Verification items for the finished model (mm, model axes). Face numbers are marked on the shaded views. A direction names the side the tool comes from. Round coordinates to 2 decimals unless told otherwise and drop trailing zeros. Order: outer loops, then holes, each group sorted by start corner. A loop starts at its lowest first (then second) coordinate and runs counter-clockwise, first axis right, second up. Notation, with made-up numbers: M 54.25,73.5 L 85.25,73.5 A4 cw 85.25,77.5 Z; hole C 8,29.25 d3. An arc over 180 degrees is marked long. Use one line per item in the form item = value. Start each with the question number.
Item 1: Thickness scan on probe 1 along Y at (x, z) = (0, 0.7); probe 2 along X at (y, z) = (0.75, 0.55); probe 3 along Z at (x, y) = (1.75, -4.5). Record the ranges inside material, lowest first. Write a range as [from, to].
Item 2: Cross-section at A-A on y = 0. Enter the section's corners in (x, z) (3 decimals).
Item 3: Cross-section at D-D on z = 0.2. Enter the section's corners in (x, y).
Item 4: Go/stop test with a flat-tipped pin: pin 1 Ø3 at (x, y) = (0, 0) entering from -Z. Record where the tip stops, or that it passes through.
Item 5: Cross-section at C-C on y = -1.5. Enter the section's corners in (x, z) (3 decimals).
Item 6: Tool access check on the marked faces 1, 2, 3, 4 and 5. Record the directions out of +Z, -Z, +X, -X, +Y, -Y that give a thin tool (end or side, any length) a straight path to the whole face; none if there is none.
Item 7: Cross-section at B-B on z = 1.75. Enter the section's corners in (x, y) (3 decimals).
from build123d import *

# Parameters (mm, degrees)
F0_R          = 5.2
F1_DEPTH      = 1
F2_R          = 2
F3_DEPTH      = 1.48
F4_DEPTH      = 25
F4_DEPTH_BACK = 25
F5_R          = 0.1


with BuildPart() as f1:
    # F0 (on Top) → F1 (new body)
    with BuildSketch(Plane.XY):
        Circle(F0_R)
    extrude(amount=F1_DEPTH)

    # F2 (on face) → F3 (join)
    with BuildSketch(Plane.XY.offset(1)):
        Polygon((3.575, -2.064027), (3.575, 2.064027), (0, 4.128054), (-3.575, 2.064027), (-3.575, -2.064027), (0, -4.128054), align=None)
        Circle(F2_R, mode=Mode.SUBTRACT)
    extrude(amount=F3_DEPTH)

    # F2 (on face) → F4 (cut, two sides)
    with BuildSketch(Plane.XY.offset(1)) as f4_sk:
        Circle(F2_R)
    extrude(amount=-F4_DEPTH, mode=Mode.SUBTRACT)
    extrude(f4_sk.sketch, amount=-F4_DEPTH_BACK, mode=Mode.SUBTRACT)

    # F5
    f5_edges = [f1.edges().sort_by_distance(p)[0] for p in [
        (1.7875, -3.096041, 2.48),
        (3.575, 0, 2.48),
        (-1.7875, -3.096041, 2.48),
        (-3.575, 0, 2.48),
        (-1.7875, 3.096041, 2.48),
        (1.7875, 3.096041, 2.48),
    ]]
    fillet(f5_edges, radius=F5_R)


solid = f1.part
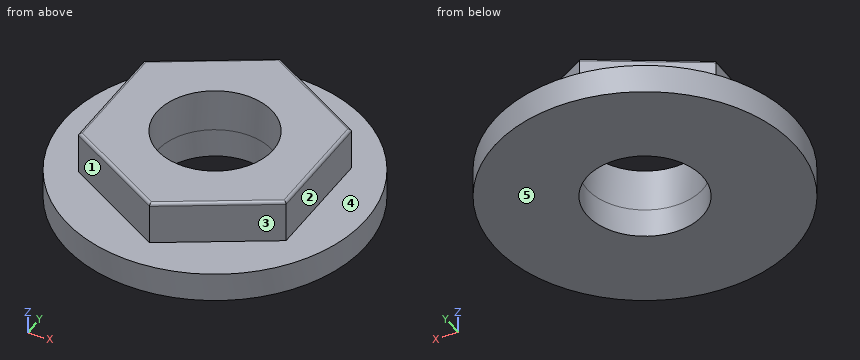
Output values:
q1.probe_1 = [-5.2, -2], [2, 5.2]
q1.probe_2 = [-5.15, -1.85], [1.85, 5.15]
q1.probe_3 = [0, 1]
q2.outline = M -5.2,0 L -2,0 L -2,2.48 L -3.475,2.48 A0.1 ccw -3.575,2.38 L -3.575,1 L -5.2,1 Z; M 2,0 L 5.2,0 L 5.2,1 L 3.575,1 L 3.575,2.38 A0.1 ccw 3.475,2.48 L 2,2.48 Z
q3.outline = C 0,0 d10.4; hole C 0,0 d4
q4.pin_1 = through
q5.outline = M -4.979,0 L -1.323,0 L -1.323,2.48 L -3.475,2.48 A0.1 ccw -3.575,2.38 L -3.575,1 L -4.979,1 Z; M 1.323,0 L 4.979,0 L 4.979,1 L 3.575,1 L 3.575,2.38 A0.1 ccw 3.475,2.48 L 1.323,2.48 Z
q6.face_1 = +Z, -X, -Y
q6.face_2 = +Z, +X, +Y, -Y
q6.face_3 = +Z, +X, -Y
q6.face_4 = +Z
q6.face_5 = -Z, +X, -X, +Y, -Y
q7.outline = M -3.575,-2.064 L 0,-4.128 L 3.575,-2.064 L 3.575,2.064 L 0,4.128 L -3.575,2.064 Z; hole C 0,0 d4
